from build123d import *

# Parameters (mm, degrees)
BOSS_EXTRUDE2_DEPTH     = 9
BOSS_EXTRUDE3_DEPTH     = 2
SKETCH3_W               = 47.18
SKETCH3_H               = 5
BOSS_EXTRUDE4_DEPTH     = 2
SKETCH5_W               = 6.35
SKETCH5_H               = 12.7
CUT_EXTRUDE1_DEPTH      = 12
CUT_EXTRUDE1_DEPTH_BACK = 10
BOSS_EXTRUDE5_START     = 8
BOSS_EXTRUDE5_DEPTH     = 10
BOSS_EXTRUDE6_START     = 8
BOSS_EXTRUDE6_DEPTH     = 10
CUT_EXTRUDE2_DEPTH      = 8


with BuildPart() as part:
    # Sketch1 → Boss-Extrude2 (new body)
    with BuildSketch(Plane(origin=(0, 0, 0), x_dir=(1, 0, 0), z_dir=(0, 1, 0))):
        Polygon((9.43, 34.38), (9.43, 61.69), (11.97, 61.69), (11.97, 66.77), (15.78, 66.77), (15.78, 76.93), (27.4, 76.93), (27.4, 66.77), (31.21, 66.77), (31.21, 61.69), (33.75, 61.69), (33.75, 34.38), (38.83, 34.38), (38.83, 14.7), (45.18, 14.7), (45.18, -2), (-2, -2), (-2, 14.7), (4.35, 14.7), (4.35, 34.38), align=None)
        Polygon((0, 0), (0, 12.7), (6.35, 12.7), (6.35, 32.38), (11.43, 32.38), (11.43, 59.69), (13.97, 59.69), (13.97, 64.77), (17.78, 64.77), (17.78, 74.93), (25.4, 74.93), (25.4, 64.77), (29.21, 64.77), (29.21, 59.69), (31.75, 59.69), (31.75, 32.38), (36.83, 32.38), (36.83, 12.7), (43.18, 12.7), (43.18, 0), align=None, mode=Mode.SUBTRACT)
    extrude(amount=BOSS_EXTRUDE2_DEPTH)

    # Sketch2 → Boss-Extrude3 (add)
    with BuildSketch(Plane(origin=(0, 9, 0), x_dir=(1, 0, 0), z_dir=(0, 1, 0))):
        Polygon((-2, -2), (-2, 14.7), (4.35, 14.7), (4.35, 34.38), (9.43, 34.38), (9.43, 61.69), (11.97, 61.69), (11.97, 66.77), (15.78, 66.77), (15.78, 76.93), (27.4, 76.93), (27.4, 66.77), (31.21, 66.77), (31.21, 61.69), (33.75, 61.69), (33.75, 34.38), (38.83, 34.38), (38.83, 14.7), (45.18, 14.7), (45.18, -2), align=None)
    extrude(amount=BOSS_EXTRUDE3_DEPTH)

    # Sketch3 → Boss-Extrude4 (add)
    with BuildSketch(Plane.XZ):
        with Locations((21.59, -0.5)):
            Rectangle(SKETCH3_W, SKETCH3_H)
    extrude(amount=BOSS_EXTRUDE4_DEPTH)

    # Sketch5 → Cut-Extrude1 (cut, two sides)
    with BuildSketch(Plane.XZ.offset(-9)) as cut_extrude1_sk:
        with Locations((40.005, -6.35)):
            Rectangle(SKETCH5_W, SKETCH5_H)
    extrude(amount=CUT_EXTRUDE1_DEPTH, mode=Mode.SUBTRACT)
    extrude(cut_extrude1_sk.sketch, amount=-CUT_EXTRUDE1_DEPTH_BACK, mode=Mode.SUBTRACT)

    # Sketch8 → Boss-Extrude5 (add)
    with BuildSketch(Plane.XY.offset(-59.69).offset(BOSS_EXTRUDE5_START)):
        Polygon((11.43, 0), (12.43, 1), (11.43, 2), (11.43, 1), align=None)
    extrude(amount=BOSS_EXTRUDE5_DEPTH)

    # Sketch9 → Boss-Extrude6 (add)
    with BuildSketch(Plane.XY.offset(-59.69).offset(BOSS_EXTRUDE6_START)):
        Polygon((31.75, 0), (31.75, 1), (31.75, 2), (30.75, 1), align=None)
    extrude(amount=BOSS_EXTRUDE6_DEPTH)

    # Sketch10 → Cut-Extrude2 (cut)
    with BuildSketch(Plane.XZ.offset(2)):
        Polygon((31.270231455, -3), (10.582199871, -3), (10.582199871, 0), (31.270231455, 0), (42.389768545, 0), (42.389768545, -6), (31.270231455, -6), align=None)
    extrude(amount=-CUT_EXTRUDE2_DEPTH, mode=Mode.SUBTRACT)


solid = part.part
Check sheet for the modelled part. Datum: model origin and axes. Units: mm. A direction names the side the tool comes from. Round coordinates to 2 decimals unless told otherwise and drop trailing zeros. Order: outer loops, then holes, each group sorted by start corner. A loop starts at its lowest first (then second) coordinate and runs counter-clockwise, first axis right, second up.
(1) Scan lines: probe 1 along X at (y, z) = (4.75, -54.5); probe 2 along X at (y, z) = (6.75, -60); probe 3 along Z at (x, y) = (5, 7.25). Record each from-to range of solid material in increasing order.
(2) Cross-section at C-C, the plane x = 8. Enter the section's corners in (y, z), and give its area (3 significant figures).
(3) Draft check along Y on faces 1 (the flat face through (31.75, 4, -46)), 2 (the flat face through (22, 11, -29)), 3 (the flat face through (6.35, 4, -22)), 4 (the flat face through (0, 4, -6)). Enter one of: pulls with the +Y half, pulls with the -Y half, needs draft (parallel to the pull), parting line crosses it, or undercut.
(4) Cross-section at A-A, the plane z = -10. Enter the section's corners in (x, y), and give its area (3 significant figures).
(5) Access from +Z, -Z, +X, -X, +Y, -Y to the whole of each face (thin tool, end or side, straight path). Record for faces 5 (the flat face through (15.78, 5, -72)), 6 (the flat face through (40, 5, -12.7)), 7 (the flat face through (31.21, 5, -64)), 8 (the flat face through (10.582, -1, -2)), 9 (the flat face through (27, 4, -64.77)).
(6) Cross-section at D-D, the plane z = -72. Enter the section's corners in (x, y), and give its area (3 significant figures).
(7) Go/stop test with flat-tipped pins: P1, Ø5.5, axis at y = 5, z = -62.5, coming from the +X side; P2, Ø0.8, axis at x = 12, y = 1, coming from the -Z side; P3, Ø5, axis at y = 3, z = -39, coming from the -X side. Record where each tip stops, or that it passes through.
(8) Cross-section at B-B, the plane x = 38. Enter the section's corners in (y, z).
Check sheet entries:
1. probe 1: x = 9.43 to 11.43, 31.75 to 33.75
1. probe 2: x = 9.43 to 13.97, 29.21 to 33.75
1. probe 3: z = -34.38 to -12.7, 0 to 2
2. outline: (-2, -3) - (0, -3) - (0, 0) - (9, 0) - (9, -32.38) - (0, -32.38) - (0, -34.38) - (11, -34.38) - (11, 2) - (-2, 2) - close
2. area: 119 mm2
3. face 1: undercut
3. face 2: pulls with the +Y half
3. face 3: needs draft
3. face 4: undercut
4. outline: (-2, 0) - (0, 0) - (0, 9) - (36.83, 9) - (36.83, 11) - (-2, 11) - close; (43.18, 0) - (45.18, 0) - (45.18, 11) - (43.18, 11) - close
4. area: 118 mm2
5. face 5: -Z, -X, +Y, -Y
5. face 6: +Y, -Y
5. face 7: -Z, +X, +Y, -Y
5. face 8: -Z, -Y
5. face 9: -Y
6. outline: (15.78, 0) - (17.78, 0) - (17.78, 9) - (25.4, 9) - (25.4, 0) - (27.4, 0) - (27.4, 11) - (15.78, 11) - close
6. area: 59.2 mm2
7. P1: stops at x = 33.75
7. P2: stops at z = -66.77
7. P3: stops at x = 9.43
8. outline: (-2, 0) - (11, 0) - (11, 2) - (-2, 2) - close; (0, -34.38) - (11, -34.38) - (11, -12.7) - (0, -12.7) - close
